Geometry: final body of the model. Coordinates: model frame, mm. A direction names the side the tool comes from. Round coordinates to 2 decimals unless told otherwise and drop trailing zeros. Loops run counter-clockwise (first coordinate to the right, second up) from the corner with the lowest first, then second, coordinate; pieces in that order, holes last. Notation, with made-up numbers: (40, 89.5) -> (77, 89.5) arc R33 ccw to (77, 120.5) -> close; hole circle Ø9 at (66.25, 20). An arc over 180 degrees is marked (long way). Answer in a Markdown table with one row per item.
```python
from build123d import *

# Parameters (mm, degrees)
F0_W     = 38
F0_H     = 48
F0_W_2   = 24
F0_H_2   = 34
F1_DEPTH = 12.5
F2_R     = 5
F4_DEPTH = 5
F5_R     = 5
F3_R     = 2.5
F6_DEPTH = 7.5
F8_DEPTH = 5


with BuildPart() as f1:
    # F0 (on Top) → F1 (new body)
    with BuildSketch(Plane.XY):
        with Locations((0, 0.012681)):
            Rectangle(F0_W, F0_H)
        with Locations((0, 0.012681)):
            Rectangle(F0_W_2, F0_H_2, mode=Mode.SUBTRACT)
        with Locations((0, 0.012681)):
            Rectangle(F0_W_2, F0_H_2)
    extrude(amount=F1_DEPTH)

    # F2
    f2_edges = [f1.edges().sort_by_distance(p)[0] for p in [
        (-19, -23.987319, 6.25),
        (19, -23.987319, 6.25),
        (19, 24.012681, 6.25),
        (-19, 24.012681, 6.25),
    ]]
    fillet(f2_edges, radius=F2_R)

    # F0 (on Top) → F4 (cut)
    with BuildSketch(Plane.XY):
        with Locations((0, 0.012681)):
            Rectangle(F0_W_2, F0_H_2)
    extrude(amount=F4_DEPTH, mode=Mode.SUBTRACT)

    # F5
    f5_edges = [f1.edges().sort_by_distance(p)[0] for p in [
        (-12, -16.987319, 2.5),
        (12, -16.987319, 2.5),
        (12, 17.012681, 2.5),
        (-12, 17.012681, 2.5),
    ]]
    fillet(f5_edges, radius=F5_R)

    # F3 (on face) → F6 (cut, through all)
    with BuildSketch(Plane.XY.offset(12.5)):
        with Locations((-5, -11.987319)):
            Circle(F3_R)
        with Locations((5, -11.987319)):
            Circle(F3_R)
    extrude(amount=-F6_DEPTH, mode=Mode.SUBTRACT)

    # F7 (on face) → F8 (cut)
    with BuildSketch(Plane(origin=(0, 0, 0), x_dir=(1, 0, 0), z_dir=(0, 0, -1))):
        with BuildLine():
            Line((14, -24.012681), (12, -12.012681))
            ThreePointArc((12, -12.012681), (10.535534, -15.548215), (7, -17.012681))
            Line((7, -17.012681), (-7, -17.012681))
            ThreePointArc((-7, -17.012681), (-10.535534, -15.548215), (-12, -12.012681))
            Line((-12, -12.012681), (-14, -24.012681))
            Line((-14, -24.012681), (14, -24.012681))
        make_face()
    extrude(amount=-F8_DEPTH, mode=Mode.SUBTRACT)


solid = f1.part
```
Item 1: Ray query, L1, parallel to X at y = 8.5, z = 4.75; L2, parallel to X at y = -12, z = 8; L3, parallel to Y at x = -5, z = 9.5. Return the intervals inside material, ascending.
Ans:
| item | result |
|---|---|
| L1 | -19 to -12, 12 to 19 |
| L2 | -19 to -7.5, -2.5 to 2.5, 7.5 to 19 |
| L3 | -23.99 to -14.49, -9.49 to 24.01 |
Item 2: Section query D-D, the plane x = 11.5. Output: boundary loops of the cut face in (y, z).
Ans:
| item | result |
|---|---|
| outline | (-23.99, 0) -> (-14.17, 0) -> (-14.17, 5) -> (24.01, 5) -> (24.01, 12.5) -> (-23.99, 12.5) -> close |
Item 3: Set-up query: faces 5 (the flat face through (0, 24.013, 9)), 6 (the flat face through (12, 0, 2)). Return all of +Z, -Z, +X, -X, +Y, -Y with unobstructed straight access to the full face (end or side cutting, diameter ignored); none if empty.
Ans:
| item | result |
|---|---|
| face 5 | +Z, -Z, +X, -X, +Y |
| face 6 | -Z, +Y |
Item 4: Section query B-B, the plane z = 6. Output: boundary loops of the cut face in (x, y).
Ans:
| item | result |
|---|---|
| outline | (-19, -18.99) arc R5 ccw to (-14, -23.99) -> (14, -23.99) arc R5 ccw to (19, -18.99) -> (19, 19.01) arc R5 ccw to (14, 24.01) -> (-14, 24.01) arc R5 ccw to (-19, 19.01) -> close; hole circle Ø5 at (-5, -11.99); hole circle Ø5 at (5, -11.99) |
Item 5: Mould query, pull axis X, two halves, no side actions, for faces 1 (the flat face through (0, -23.987, 6)), 2 (the flat face through (-19, 0, 6)), 3 (the cylindrical face through (-2.615, -11.236, 8.802)), 4 (the cylindrical face through (17.574, 22.509, 6.338)). Classes: released by +X, released by -X, zero draft, split by the parting line, or undercut.
Ans:
| item | result |
|---|---|
| face 1 | zero draft |
| face 2 | released by -X |
| face 3 | undercut |
| face 4 | released by +X |
Item 6: Section query A-A, the plane x = -5. Output: boundary loops of the cut face in (y, z).
Ans:
| item | result |
|---|---|
| outline | (-23.99, 0) -> (-16.99, 0) -> (-16.99, 5) -> (-14.49, 5) -> (-14.49, 12.5) -> (-23.99, 12.5) -> close; (-9.49, 5) -> (24.01, 5) -> (24.01, 12.5) -> (-9.49, 12.5) -> close |
Item 7: Section query C-C, the plane y = -3.5. Output: boundary loops of the cut face in (x, z).
Ans:
| item | result |
|---|---|
| outline | (-19, 0) -> (-12, 0) -> (-12, 5) -> (12, 5) -> (12, 0) -> (19, 0) -> (19, 12.5) -> (-19, 12.5) -> close |
Item 8: First-contact query: P1, Ø6.5, axis at x = 5, y = -11.99, coming from the -Z side; P2, Ø6.5, axis at x = -5, y = -11.99, coming from the +Z side; P3, Ø1, axis at x = -15, z = 6, coming from the -Y side; P4, Ø5.5, axis at x = 3.5, z = 2, coming from the +Y side. Flat tips, straight axial feed; report the tip coordinate or a pass-through.
Ans:
| item | result |
|---|---|
| P1 | z = 5 |
| P2 | z = 12.5 |
| P3 | y = -23.96 |
| P4 | y = -16.99 |
